Build history of the part. All positions in model axes, mm. A direction names the side the tool comes from. Give positions to 0.01 mm unless a question says otherwise; leave off trailing zeros. Order: outer loops, then holes, each group sorted by start corner. A loop starts at its lowest first (then second) coordinate and runs counter-clockwise, first axis right, second up. Notation, with made-up numbers: (33.25, 51.5) -> (67.25, 51.5) arc R12 cw to (67.25, 71.5) -> close; hole circle Ø5 at (-22, 70.25). An arc over 180 degrees is marked (long way). Use a Markdown table: item, result. Add a question column.
```python
from build123d import *

# Parameters (mm, degrees)
F0_R     = 1.65
F1_DEPTH = 2


with BuildPart() as f1:
    # F0 (on Right) → F1 (new body)
    with BuildSketch(Plane.YZ):
        with BuildLine():
            Line((-29, 0), (-31, 0))
            Line((-31, 0), (-31, 4))
            Line((-31, 4), (-31, 19.617821))
            ThreePointArc((-31, 19.617821), (-60.66964, 14.832498), (-64.304047, -15))
            Line((-64.304047, -15), (-42.653412, -15))
            Line((-42.653412, -15), (-29, -15))
            Line((-29, -15), (-29, -17))
            Line((-29, -17), (-25.5, -17))
            Line((-25.5, -17), (-25.5, -15))
            Line((-25.5, -15), (-23.5, -15))
            Line((-23.5, -15), (-23.5, 0))
            Line((-23.5, 0), (-25.5, 0))
            Line((-25.5, 0), (-25.5, 4))
            Line((-25.5, 4), (-29, 4))
            Line((-29, 4), (-29, 0))
        make_face()
        with Locations((-42.653412, -2.5)):
            Circle(F0_R, mode=Mode.SUBTRACT)
    extrude(amount=F1_DEPTH)


solid = f1.part
```
(1) Pin check, flat tips, straight feed: pin 1 Ø0.6 at (x, z) = (1, -15.5) entering from -Y; pin 2 Ø1 at (x, z) = (1.5, 1.5) entering from +Y; pin 3 Ø1 at (x, y) = (1.5, -24) entering from +Z. Stop position of each tip, or through.
(2) Band-saw the part on B-B on x = 0.6. Give the cut face in (y, z).
(3) Mould opens along Z. For faces 5 (the face through (1, -44.3, -2.4)), 6 (the face through (1, -47, -15)), 7 (the face through (1, -25.5, 2)) say: released by +Z, released by -Z, zero draft, split by the parting line, or undercut.
(4) Band-saw the part on A-A on z = -2.5. Give the cut face in (x, y), plus the area to 3 significant figures.
(5) Band-saw the part on C-C on z = 11. Give the cut face in (x, y).
(6) Band-saw the part on D-D on y = -33.5. Give the cut face in (x, z).
(7) Tool access for faces 1 (the face through (1, -29, -16)), 2 (the face through (1, -25.5, -16)), 3 (the face through (1, -29, 2)), 4 (the face through (1, -27, 4)): list every direction of +Z, -Z, +X, -X, +Y, -Y with a clear straight run to the whole face (end or side of a thin tool).
(8) Wall check: probe 1 along Z at (x, y) = (1.2, -30); probe 2 along Z at (x, y) = (1.95, -27.5); probe 3 along Z at (x, y) = (1, -41.5). Give the ranges that are in metal, low to high.
Response:
| question | item | result |
|---|---|---|
| 1 | pin 1 | stops at y = -29 |
| 1 | pin 2 | stops at y = -25.5 |
| 1 | pin 3 | stops at z = 0 |
| 2 | outline | (-64.3, -15) -> (-29, -15) -> (-29, -17) -> (-25.5, -17) -> (-25.5, -15) -> (-23.5, -15) -> (-23.5, 0) -> (-25.5, 0) -> (-25.5, 4) -> (-29, 4) -> (-29, 0) -> (-31, 0) -> (-31, 19.62) arc R25 ccw to start; hole circle Ø3.3 at (-42.65, -2.5) |
| 3 | face 5 | undercut |
| 3 | face 6 | released by -Z |
| 3 | face 7 | zero draft |
| 4 | outline | (0, -67.65) -> (2, -67.65) -> (2, -44.3) -> (0, -44.3) -> close; (0, -41) -> (2, -41) -> (2, -23.5) -> (0, -23.5) -> close |
| 4 | area | 81.7 mm² |
| 5 | outline | (0, -63.7) -> (2, -63.7) -> (2, -31) -> (0, -31) -> close |
| 6 | outline | (0, -15) -> (2, -15) -> (2, 20.76) -> (0, 20.76) -> close |
| 7 | face 1 | -Z, +X, -X, -Y |
| 7 | face 2 | -Z, +X, -X, +Y |
| 7 | face 3 | +Z, +X, -X |
| 7 | face 4 | +Z, +X, -X, +Y |
| 8 | probe 1 | z = -15 to 0 |
| 8 | probe 2 | z = -17 to 4 |
| 8 | probe 3 | z = -15 to -3.68, -1.32 to 22.47 |
